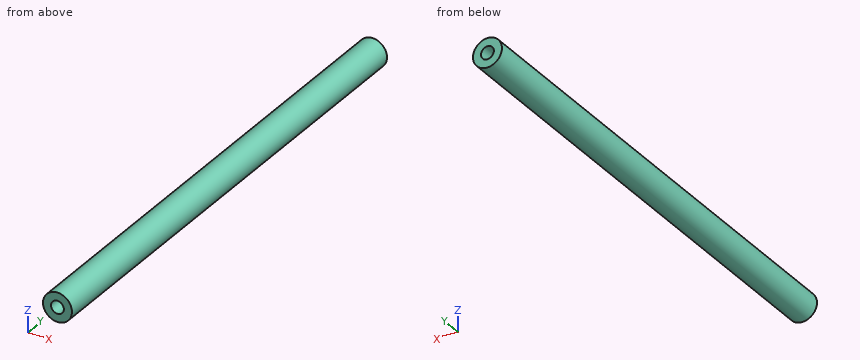
Autodesk Inventor part; units mm, degrees
ref_plane "YZ Plane" through (0, 0, 0) normal (1, 0, 0) x (0, 1, 0)
ref_plane "XZ Plane" through (0, 0, 0) normal (0, 1, 0) x (-1, 0, 0)
ref_plane "XY Plane" through (0, 0, 0) normal (0, 0, 1) x (1, 0, 0)
sketch "Sketch1" plane through (0, 0, 0) normal (0, 1, 0) x (-1, 0, 0)
  circle A0 centre (0, 0) radius 7.5
  dimension "d0" = 15
extrude "Extrusion1" add sketch "Sketch1" along normal blind 260
sketch "Sketch2" plane through (0, 260, 0) normal (0, 1, 0) x (1, 0, 0)
  point P0 (0, 0)
  point P1 (0, 0)
hole "Hole1" at (0, 260, 0) direction (0, -1, 0) diameter 6.647 depth 22.2 tip angle 118
sketch "Sketch3" plane through (0, 0, 0) normal (0, -1, 0) x (1, 0, 0)
  point P0 (0, 0)
  point P1 (0, 0)
hole "Hole2" at (0, 0, 0) direction (0, 1, 0) diameter 6.647 depth 22.2 tip angle 118
properties part number "Structure_bar"
Geometry check sheet. Reference: the model listing, model coordinates, mm. Give positions to 0.01 mm unless a question says otherwise; leave off trailing zeros. Loops run counter-clockwise (first coordinate to the right, second up) from the corner with the lowest first, then second, coordinate; pieces in that order, holes last. Notation, with made-up numbers: (-10.5, 71) - (3.5, 71) arc R23 cw to (3.5, 94) - close; hole circle Ø2 at (63, 49). An arc over 180 degrees is marked (long way). Use CSV: the item, a comma, the result in double quotes. Start each with the question number.
Q1. Section check A-A, the plane y = 232.5. Record the cut outline in (x, z).
Q2. Scan lines: probe 1 along Z at (x, y) = (0, 249); probe 2 along Z at (x, y) = (0.25, 188); probe 3 along Y at (x, z) = (0.25, 3.25). Record each from-to range of solid material in increasing order. Write a range as from..to.
Q3. Go/stop test with flat-tipped pins: pin 1 Ø1 at (y, z) = (198.5, -5) entering from -X; pin 2 Ø6 at (y, z) = (48.5, -4) entering from -X; pin 3 Ø6 at (x, z) = (0, 0) entering from +Y. Record where each tip stops, or that it passes through.
Findings below:
1,outline,"circle Ø15 at (0, 0)"
2,probe 1,"z = -7.5..-3.32, 3.32..7.5"
2,probe 2,"z = -7.5..7.5"
2,probe 3,"y = 22.24..237.76"
3,pin 1,"stops at x = -6"
3,pin 2,"stops at x = -7.43"
3,pin 3,"stops at y = 237.61"
